Autodesk Inventor part; units mm, degrees
ref_plane "YZ Plane" through (0, 0, 0) normal (1, 0, 0) x (0, 1, 0)
ref_plane "XZ Plane" through (0, 0, 0) normal (0, 1, 0) x (-1, 0, 0)
ref_plane "XY Plane" through (0, 0, 0) normal (0, 0, 1) x (1, 0, 0)
sketch "Sketch12" plane through (0, 0, 0) normal (0, 0, 1) x (1, 0, 0)
  circle A0 centre (0, 0) radius 12.5
  dimension "d22" = 25
extrude "Extrusion3" add sketch "Sketch12" along normal blind 50
sketch "Sketch15" plane through (0, 0, 50) normal (0, 0, 1) x (1, 0, 0)
  circle A0 centre (0, 0) radius 12.5
  line L0 (-5.6199, 11.1654) -> (6.24, 11.1654)
  line L1 (6.24, 11.1654) -> (6.24, 16.8143)
  line L2 (6.24, 16.8143) -> (-5.6199, 16.8143)
  line L3 (-5.6199, 16.8143) -> (-5.6199, 11.1654)
extrude "Extrusion4" cut sketch "Sketch15" against normal blind 64.3 contours L3 L2 L1 L0 A0 | A0 L0 picked at (0.9627, 11.4975)
sketch "Sketch17" plane through (-5.6199, 11.1654, 50) normal (0, 1, 0) x (1, 0, 0)
  point P0 (5.6199, 50)
sketch "Sketch18" plane through (-5.6199, 11.1654, 50) normal (0, 1, 0) x (1, 0, 0)
  line L0 (-1.8801, 28.4) -> (13.1199, 28.4)
  line L1 (13.1199, 28.4) -> (13.1199, 21.6)
  line L2 (13.1199, 21.6) -> (-1.8801, 21.6)
  line L3 (-1.8801, 21.6) -> (-1.8801, 28.4)
  line L4 (-1.8801, 28.4) -> (13.1199, 21.6) construction
  line L5 (13.1199, 28.4) -> (-1.8801, 21.6) construction
  point P0 (5.6199, 50)
  point P1 (5.6199, 25)
  dimension "d30" = 15
  dimension "d31" = 6.8
extrude "Extrusion6" cut sketch "Sketch18" against normal blind 28.2625
properties part number "foot"
Can you work these out from the model? Positions are in its coordinate system, mm. A direction names the side the tool comes from. Coordinates: 2 decimals unless noted, no trailing zeros. Write each loop counter-clockwise with the first axis right and the second up, starting at its lowest first coordinate (ties: lowest second). Pieces come first, ordered by that corner, then holes. Notation, with made-up numbers: M -32,57 L 17,57 A32 cw 17,96 Z; hole C 35,36.5 d6. An arc over 180 degrees is marked long. Use one line per item in the form item = value.
Q1. I need wall thicknesses on line 1 along Z through (x, y) = (-6.5, 7); line 2 along Y through (x, z) = (-1.25, 15); line 3 along Y through (x, z) = (11, 20). Which ranges of each line are inside material? Lowest first, please. Write a range as from..to.
Model answer:
line_1 = 0..21.6, 28.4..50
line_2 = -12.44..11.17
line_3 = -5.94..5.94
Q2. If we section it at D-D (z = 23): Write out the boundary of the cut face in (x, y), then the cut area to 3 significant figures.
Model answer:
outline = M -7.5,-10 L -7.5,10 A12.5 ccw Z; M 7.5,-10 A12.5 ccw 7.5,10 Z
area = 140 mm^2
Q3. For P1, Ø1.5, axis at x = 2, z = 6, coming from the -Y side; P2, Ø10, axis at y = 7, z = 27.5, coming from the -X side; P3, Ø1, axis at y = 8.5, z = 15.5, coming from the -X side, each with a flat end and sliding along its axis, tell me the tip position at first contact or that it passes through.
Model answer:
P1 = -12.44
P2 = -12.34
P3 = -9.6
Q4. We'd pull the mould along X, two halves only. Please class faces 1 (the flat face through (-7.5, 0, 25)), 2 (the flat face through (0, -1, 0)), 3 (the cylindrical face through (11.766, -4.22, 24.65)): +X half, -X half, draft (parallel to the pull), parting line (faces both ways), or undercut.
Model answer:
face_1 = undercut
face_2 = draft
face_3 = parting line
Q5. If we section it at C-C (y = -10.75): Write out the boundary of the cut face in (x, z).
Model answer:
outline = M -6.38,0 L 6.38,0 L 6.38,21.6 L -6.38,21.6 Z; M -6.38,28.4 L 6.38,28.4 L 6.38,50 L -6.38,50 Z
Q6. For faces 4 (the flat face through (0, 11.165, 39)), 5 (the flat face through (7.5, 0, 25)), which set-ups out of +Z, -Z, +X, -X, +Y, -Y let a thin tool reach every point of the face, with its end or its side?
Model answer:
face_4 = +Z, -Z, +X, -X, +Y
face_5 = +Y, -Y
Q7. If we section it at B-B (x = 0): Write out the boundary of the cut face in (y, z), then the cut area to 3 significant figures.
Model answer:
outline = M -12.5,0 L 11.17,0 L 11.17,21.6 L -12.5,21.6 Z; M -12.5,28.4 L 11.17,28.4 L 11.17,50 L -12.5,50 Z
area = 1,020 mm^2
Q8. If we section it at A-A (y = 0): Write out the boundary of the cut face in (x, z), then the cut area to 3 significant figures.
Model answer:
outline = M -12.5,0 L 12.5,0 L 12.5,50 L -12.5,50 Z; hole M -7.5,21.6 L 7.5,21.6 L 7.5,28.4 L -7.5,28.4 Z
area = 1,150 mm^2
